Work out the finished part from the listing and answer in its coordinate system (mm). Face numbers are marked on the shaded views. A direction names the side the tool comes from. Round coordinates to 2 decimals unless told otherwise and drop trailing zeros. Loops run counter-clockwise (first coordinate to the right, second up) from the corner with the lowest first, then second, coordinate; pieces in that order, holes last.
```python
from build123d import *

# Parameters (mm, degrees)
F0_R     = 12
F1_DEPTH = 15
F3_DEPTH = 5
F5_DEPTH = 5


with BuildPart() as f1:
    # F0 (on Front) → F1 (new body)
    with BuildSketch(Plane.XZ):
        Circle(F0_R)
    extrude(amount=F1_DEPTH)

    # F2 (on face) → F3 (cut)
    with BuildSketch(Plane.XZ.offset(15)):
        Polygon((5.294932, 2.301527), (0.654286, 5.736309), (-4.640647, 3.434783), (-5.294932, -2.301527), (-0.654286, -5.736309), (4.640647, -3.434783), align=None)
    extrude(amount=-F3_DEPTH, mode=Mode.SUBTRACT)

    # F4 (on face) → F5 (cut)
    with BuildSketch(Plane(origin=(0, 0, 0), x_dir=(-1, 0, 0), z_dir=(0, 1, 0))):
        Polygon((6.274529, 5.095451), (-1.275526, 7.981627), (-7.550054, 2.886176), (-6.274529, -5.095451), (1.275526, -7.981627), (7.550054, -2.886176), align=None)
    extrude(amount=-F5_DEPTH, mode=Mode.SUBTRACT)


solid = f1.part
```
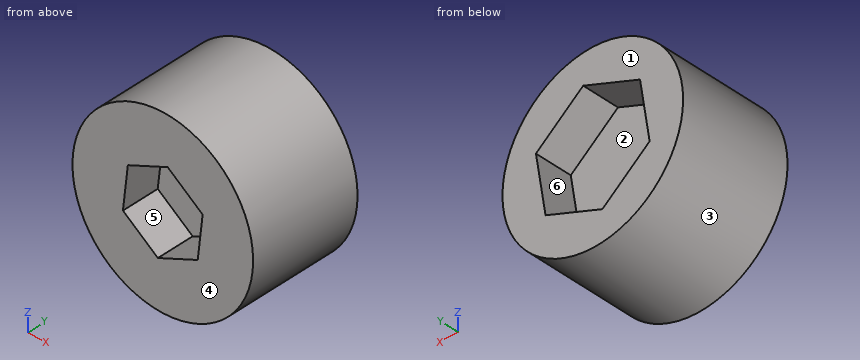
1. Determine the mould class of the marked faces 1, 2 and 3 for opening direction X: +X half, -X half, draft (parallel to the pull), parting line (faces both ways), or undercut.
Answer key:
face 1: draft
face 2: undercut
face 3: parting line
2. Which of the six approach directions +Z, -Z, +X, -X, +Y, -Y give full straight-line access (tool end or side, diameter ignored) to the marked faces 4, 5 and 6?
Answer key:
face 4: +Z, -Z, +X, -X, -Y
face 5: -Y
face 6: +Y
3. Given pin 1 (1 mm diameter, centred on y = -6, z = 6.5, fed in from +X); pin 2 (2 mm diameter, centred on x = 2, z = -0.5, fed in from +Y); pin 3 (3 mm diameter, centred on x = -2, z = 1, fed in from -Y), each flat-ended and moving along its own axis, determine where each tip first touches the part or whether it passes through.
Answer key:
pin 1: stops at x = 10.39
pin 2: stops at y = -5
pin 3: stops at y = -10
4. Find section C-C (z = 7.5). Write down the section's boundary in (x, y).
Answer key:
outline: (-9.37, -15) - (9.37, -15) - (9.37, 0) - (1.87, 0) - (1.87, -5) - (0.02, -5) - (0.02, 0) - (-9.37, 0) - close
5. Find section D-D (y = -6). Write down the section's boundary in (x, z).
Answer key:
outline: circle Ø24 at (0, 0)
6. Find section A-A (y = -12). Write down the section's boundary in (x, z).
Answer key:
outline: circle Ø24 at (0, 0); hole (-5.29, -2.3) - (-0.65, -5.74) - (4.64, -3.43) - (5.29, 2.3) - (0.65, 5.74) - (-4.64, 3.43) - close
7. Find section B-B (x = -6.75). Write down the section's boundary in (y, z), then the cut area to 3 significant figures.
Answer key:
outline: (-15, -9.92) - (0, -9.92) - (0, -3.54) - (-5, -3.54) - (-5, 2.12) - (0, 2.12) - (0, 9.92) - (-15, 9.92) - close
area: 269 mm2
8. Consider probe 1 along Y at (x, z) = (1.75, 5.5); probe 2 along X at (y, z) = (-1.5, 0.5); probe 3 along X at (y, z) = (-11.75, -1.5). Determine where each line is inside the solid, lowest interval first.
Answer key:
probe 1: y = -15 to -5
probe 2: x = -11.99 to -7.01, 7.17 to 11.99
probe 3: x = -11.91 to -5.2, 4.86 to 11.91
